from build123d import *

# Parameters (mm, degrees)
SCHIZZO3_W                   = 15
SCHIZZO3_H                   = 45
ESTRUSIONE_ESTRUSIONE1_DEPTH = 25


with BuildPart() as part:
    # Schizzo1 → Rivoluzione1 (revolve)
    with BuildSketch(Plane.XY):
        Polygon((20, 68), (109, 68), (109, 30), (30, 30), (30, 5), (48, 5), (48, 0), (0, 0), (0, 148), (20, 148), align=None)
    revolve(axis=Axis((0, -1000, 0), (0, 1, 0)))

    # Schizzo3 → Estrusione-Estrusione1 (add)
    with BuildSketch(Plane.XZ.offset(-30)):
        with Locations((0, 22.5)):
            Rectangle(SCHIZZO3_W, SCHIZZO3_H)
    extrude(amount=ESTRUSIONE_ESTRUSIONE1_DEPTH)


solid = part.part
For this review, take the finished solid that the model builds, in its own axes (mm). A direction names the side the tool comes from. Give positions to 0.01 mm unless a question says otherwise; leave off trailing zeros. Write each loop counter-clockwise with the first axis right and the second up, starting at its lowest first coordinate (ties: lowest second). Pieces come first, ordered by that corner, then holes. Notation, with made-up numbers: (-15.5, 63) -> (17.5, 63) arc R19 ccw to (17.5, 82) -> close; hole circle Ø4 at (43, 15). An arc over 180 degrees is marked (long way). Use CSV: the item, a comma, the result in double quotes.
Q1. Tool access review of faces 5 (the face through (-4.336, 107.44, 19.524)), 6 (the face through (0, 18, 45)), 7 (the face through (-7.5, 18, 37)), 8 (the face through (1.213, 17.325, -29.975)), 9 (the face through (-47.954, 2.465, -2.11)): name each direction out of +Z, -Z, +X, -X, +Y, -Y from which nothing blocks a thin tool from reaching the whole face with its end or side.
Conclusion:
face 5,"+Y"
face 6,"+Z, +X, -X"
face 7,"+Z, -X"
face 8,"none"
face 9,"-Y"
Q2. Take a section at B-B, the plane x = 0. Write out the cut boundary in (y, z).
Conclusion:
outline,"(0, -48) -> (5, -48) -> (5, -30) -> (30, -30) -> (30, -109) -> (68, -109) -> (68, -20) -> (148, -20) -> (148, 20) -> (68, 20) -> (68, 109) -> (30, 109) -> (30, 45) -> (5, 45) -> (5, 48) -> (0, 48) -> close"
Q3. To check wall thickness, follow probe 1 along Y at (x, z) = (26, 59); probe 2 along X at (y, z) = (45.5, -37.5); probe 3 along Z at (x, y) = (-88, 35.5). State the ranges of each line that lie inside material, in increasing order. Write a range as [from, to].
Conclusion:
probe 1,"[30, 68]"
probe 2,"[-102.35, 102.35]"
probe 3,"[-64.32, 64.32]"
Q4. Mouldability with a two-part tool opening along Y and no side actions: class faces 1 (the face through (-86.5, 48.73, 66.32)), 2 (the face through (-1, 0, -1)), 3 (the face through (7.5, 18, 37)), 4 (the face through (-21, 5, -22)) as pulls with the +Y half, pulls with the -Y half, needs draft (parallel to the pull), parting line crosses it, or undercut.
Conclusion:
face 1,"needs draft"
face 2,"pulls with the -Y half"
face 3,"undercut"
face 4,"undercut"
Q5. Take a section at A-A, the plane z = 0. Write out the cut boundary in (x, y).
Conclusion:
outline,"(-109, 30) -> (-30, 30) -> (-30, 5) -> (-48, 5) -> (-48, 0) -> (48, 0) -> (48, 5) -> (30, 5) -> (30, 30) -> (109, 30) -> (109, 68) -> (20, 68) -> (20, 148) -> (-20, 148) -> (-20, 68) -> (-109, 68) -> close"
Q6. Take a section at C-C, the plane y = 106. Write out the cut boundary in (x, z).
Conclusion:
outline,"circle Ø40 at (0, 0)"
Q7. For P1, Ø17.5, axis at y = 13, z = 37.5, coming from the -X side; P2, Ø3, axis at y = 38, z = 61.5, coming from the -X side; P3, Ø8, axis at x = -31, z = -65.5, coming from the +Y side, all flat-tipped, find the tip position at first contact; note any pin that passes through.
Conclusion:
P1,"x = -33.93"
P2,"x = -91"
P3,"y = 68"
Q8. Take a section at D-D, the plane y = 26. Write out the cut boundary in (x, z), then the cut area to 3 significant figures.
Conclusion:
outline,"(-7.5, 29.05) arc R30 ccw (long way) to (7.5, 29.05) -> (7.5, 45) -> (-7.5, 45) -> close"
area,"3,060 mm2"
